Autodesk Inventor part; units mm, degrees
ref_plane "YZ Plane" through (0, 0, 0) normal (1, 0, 0) x (0, 1, 0)
ref_plane "XZ Plane" through (0, 0, 0) normal (0, 1, 0) x (-1, 0, 0)
ref_plane "XY Plane" through (0, 0, 0) normal (0, 0, 1) x (1, 0, 0)
sketch "Sketch1" plane through (0, 0, 0) normal (0, 1, 0) x (-1, 0, 0)
  line L0 (-10, 2.5) -> (10, 2.5)
  line L1 (10, 2.5) -> (10, -2.5)
  line L2 (10, -2.5) -> (-10, -2.5)
  line L3 (-10, -2.5) -> (-10, 2.5)
  line L4 (-10, 2.5) -> (10, -2.5) construction
  line L5 (10, 2.5) -> (-10, -2.5) construction
  line L6 (10, 1) -> (2, 1)
  line L7 (2, 1) -> (2, -1)
  line L8 (2, -1) -> (10, -1)
  line L9 (10, -1) -> (10, 1)
  circle A0 centre (-30, 0) radius 5
  arc A1 (-10, -2.5) -> (-28.7692, -4.8462) centre (-10, -78.75) ccw
  arc A2 (-28.7692, 4.8462) -> (-10, 2.5) centre (-10, 78.75) ccw
  point P0 (0, 0)
  point P1 (0, 0)
  point P2 (2, 0)
  point P3 (0, 0)
  dimension "d0" = 5
  dimension "d1" = 20
  dimension "d2" = 8
  dimension "d3" = 2
  dimension "d6" = 10
  dimension "d7" = 30
extrude "Extrusion1" add sketch "Sketch1" along normal mid plane 5 contours L0 L1 L6 L7 L8 L2 L3 | L3 A1 A0 A2 | A0
sketch "Sketch3" plane through (0, 2.5, 0) normal (0, 1, 0) x (1, 0, 0)
  arc A0 (28.7692, -4.8462) -> (28.7692, -4.8462) centre (30, 0) ccw
  point P0 (0, 0)
  point P1 (37.473, -9.6754)
  point P2 (37.473, 9.6754)
  point P3 (23.4247, 7.5342)
hole "Hole1" at (30, 2.5, 0) direction (0, -1, 0) diameter 4.496 end through all
properties part number "ChipPusher"
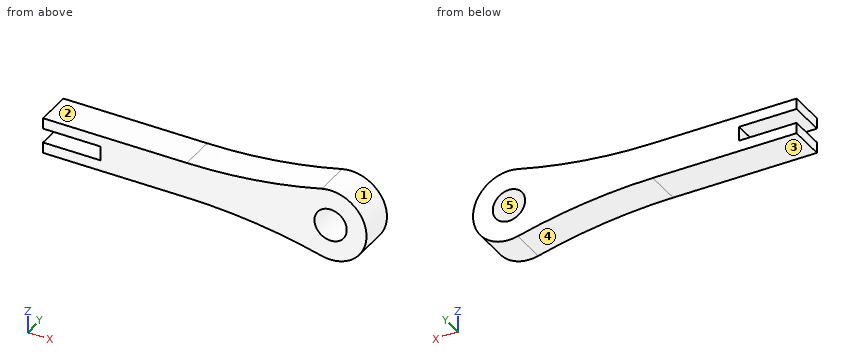
The listing builds one solid part. Answer for the finished solid, in the listing's coordinates (mm). Face numbers are marked on the shaded views. A direction names the side the tool comes from. Give positions to 0.01 mm unless a question says otherwise; leave off trailing zeros. Order: outer loops, then holes, each group sorted by start corner. A loop starts at its lowest first (then second) coordinate and runs counter-clockwise, first axis right, second up.
1) Given P1, Ø1.5, axis at x = -4, y = -1, coming from the +Z side; P2, Ø1.5, axis at x = -6, y = 1, coming from the -Z side, each flat-ended and moving along its own axis, determine where each tip first touches the part or whether it passes through.
Reported:
P1: stops at z = 2.5
P2: stops at z = -2.5
2) Consider line 1 along Z through (x, y) = (30, 0.9); line 2 along Z through (x, y) = (-6, -2.1); line 3 along Z through (x, y) = (5.5, 1.3). Determine where each line is inside the solid, lowest interval first.
Reported:
line 1: z = -5 to -2.25, 2.25 to 5
line 2: z = -2.5 to -1, 1 to 2.5
line 3: z = -2.5 to 2.5
3) Find section D-D on x = 0. Write down the section's boundary in (y, z), then the cut area to 3 significant figures.
Reported:
outline: (-2.5, -2.5) - (2.5, -2.5) - (2.5, 2.5) - (-2.5, 2.5) - close
area: 25.0 mm2
4) Find section C-C on y = 1.15. Write down the section's boundary in (x, z), then the cut area to 3 significant figures.
Reported:
outline: (-10, -2.5) - (10, -2.5) arc R76.25 cw to (28.77, -4.85) arc R5 ccw (long way) to (28.77, 4.85) arc R76.25 cw to (10, 2.5) - (-10, 2.5) - (-10, 1) - (-2, 1) - (-2, -1) - (-10, -1) - close; hole circle Ø4.5 at (30, 0)
area: 243 mm2
5) Determine the mould class of the marked faces 3, 4 and 5 for opening direction X: pulls with the +X half, pulls with the -X half, needs draft (parallel to the pull), parting line crosses it, or undercut.
Reported:
face 3: needs draft
face 4: pulls with the -X half
face 5: undercut
6) For the marked faces 1 and 2, determine the directions among +Z, -Z, +X, -X, +Y, -Y from which every point of the face is accessible in a straight line to the end or side of a thin tool.
Reported:
face 1: +Y, -Y
face 2: +Z, -X, +Y, -Y
7) Find section B-B on x = 30. Write down the section's boundary in (y, z), then the cut area to 3 significant figures.
Reported:
outline: (-2.5, -5) - (2.5, -5) - (2.5, -2.25) - (-2.5, -2.25) - close; (-2.5, 2.25) - (2.5, 2.25) - (2.5, 5) - (-2.5, 5) - close
area: 27.5 mm2
8) Find section A-A on z = 0. Write down the section's boundary in (x, y), then the cut area to 3 significant figures.
Reported:
outline: (-2, -2.5) - (27.75, -2.5) - (27.75, 2.5) - (-2, 2.5) - close; (32.25, -2.5) - (35, -2.5) - (35, 2.5) - (32.25, 2.5) - close
area: 163 mm2
